```python
from build123d import *

# Parameters (mm, degrees)
SKETCH1_R               = 20
SKETCH1_R_2             = 1.475
BOSS_EXTRUDE1_DEPTH     = 6
CUT_EXTRUDE1_REACH      = 30.914
CUT_EXTRUDE1_END_RADIUS = 20
SKETCH2_R               = 1.975


with BuildPart() as part:
    # Sketch1 → Boss-Extrude1 (new body)
    # profile 1 of 2: a face of its own
    with BuildSketch(Plane.XY):
        Circle(SKETCH1_R)
        with Locations((-10.606601718, -10.606601718)):
            Circle(SKETCH1_R_2, mode=Mode.SUBTRACT)
        with Locations((10.606601718, -10.606601718)):
            Circle(SKETCH1_R_2, mode=Mode.SUBTRACT)
        with Locations((-10.606601718, 10.606601718)):
            Circle(SKETCH1_R_2, mode=Mode.SUBTRACT)
        with BuildLine():
            ThreePointArc((4.125, 0), (-1.684302549, -3.765468088), (-2.749545417, 3.075))
            ThreePointArc((-2.749545417, 3.075), (0, 4.125), (2.749545417, 3.075))
            ThreePointArc((2.749545417, 3.075), (3.765468088, 1.684302549), (4.125, 0))
        make_face(mode=Mode.SUBTRACT)
        with Locations((10.606601718, 10.606601718)):
            Circle(SKETCH1_R_2, mode=Mode.SUBTRACT)
    # profile 2 of 2: a face of its own
    with BuildSketch(Plane.XY):
        with BuildLine():
            ThreePointArc((2.749545417, 3.075), (0, 4.125), (-2.749545417, 3.075))
            Line((-2.749545417, 3.075), (2.749545417, 3.075))
        make_face()
    extrude(amount=BOSS_EXTRUDE1_DEPTH)

    # Cut-Extrude1: up to this cylinder (the profile starts inside it)
    cut_extrude1_end = Plane(origin=(0, 0, 3), z_dir=(0, 0, -1)) * Cylinder(CUT_EXTRUDE1_END_RADIUS, 102.828, mode=Mode.PRIVATE)
    # Sketch2 → Cut-Extrude1 (cut, up to the surface)
    with BuildSketch(Plane(origin=(0, 0, 0), x_dir=(1, 0, 0), z_dir=(0, 1, 0)), mode=Mode.PRIVATE) as cut_extrude1_sk1:
        with Locations(Location((0, -3, 0), (0, 0, 90))):
            Circle(SKETCH2_R)
    cut_extrude1_tool1 = extrude(cut_extrude1_sk1.sketch, amount=CUT_EXTRUDE1_REACH, mode=Mode.PRIVATE) & cut_extrude1_end
    add(cut_extrude1_tool1.solids().sort_by_distance((0, 0, 3))[0], mode=Mode.SUBTRACT)


solid = part.part
```
Design review of the part built by this model. Coordinates are the model's own, in mm. A direction names the side the tool comes from. Coordinates: 2 decimals unless noted, no trailing zeros. Loops run counter-clockwise (first coordinate to the right, second up) from the corner with the lowest first, then second, coordinate; pieces in that order, holes last.
Q1. For pin 1 (2.5 mm diameter, centred on x = 0, z = 2, fed in from -Y); pin 2 (1 mm diameter, centred on y = 5, z = 2.5, fed in from +X); pin 3 (3.5 mm diameter, centred on x = 0, z = 3, fed in from +Y), all flat-tipped, find the tip position at first contact; note any pin that passes through.
Reported:
pin 1: stops at y = -20
pin 2: stops at x = 19.49
pin 3: stops at y = -3.74
Q2. We need section B-B on z = 4. State the section outline as (x, y) points (3 decimals), and give its area (3 significant figures).
Reported:
outline: (-2.75, 3.075) - (-1.703, 3.075) - (-1.703, 19.927) arc R20 ccw (long way) to (1.703, 19.927) - (1.703, 3.075) - (2.75, 3.075) arc R4.125 cw (long way) to start; hole circle Ø2.95 at (-10.607, -10.607); hole circle Ø2.95 at (-10.607, 10.607); hole circle Ø2.95 at (10.607, -10.607); hole circle Ø2.95 at (10.607, 10.607)
area: 1,120 mm2
Q3. We need section D-D on x = -16. State the section outline as (y, z) points.
Reported:
outline: (-12, 0) - (12, 0) - (12, 6) - (-12, 6) - close
Q4. To check wall thickness, follow line 1 (Y direction, x = 11.5, z = 4); line 2 (X direction, y = 9.5, z = 5.75); line 3 (Y direction, x = 11, z = 2.75). State the ranges of each line that lie inside material, in increasing order.
Reported:
line 1: y = -16.36 to -11.78, -9.43 to 9.43, 11.78 to 16.36
line 2: x = -17.6 to -11.58, -9.63 to 9.63, 11.58 to 17.6
line 3: y = -16.7 to -12.03, -9.19 to 9.19, 12.03 to 16.7
Q5. We need section C-C on y = 14. State the section outline as (x, z) points (3 decimals).
Reported:
outline: (-14.283, 0) - (14.283, 0) - (14.283, 6) - (-14.283, 6) - close; hole circle Ø3.95 at (0, 3)
Q6. Tool access review of faces 5 (the face through (0, 5, 0)), 6 (the face through (-2, 3.075, 2)), 7 (the face through (1.2, 11.42, 4.57)): name each direction out of +Z, -Z, +X, -X, +Y, -Y from which nothing blocks a thin tool from reaching the whole face with its end or side.
Reported:
face 5: -Z, +X, -X, +Y, -Y
face 6: +Z, -Z
face 7: +Y
Q7. We need section A-A on x = 0. State the section outline as (y, z) points (3 decimals), and give its area (3 significant figures).
Reported:
outline: (-20, 0) - (-4.125, 0) - (-4.125, 6) - (-20, 6) - close; (3.075, 0) - (20, 0) - (20, 1.025) - (3.075, 1.025) - close; (3.075, 4.975) - (20, 4.975) - (20, 6) - (3.075, 6) - close
area: 130 mm2
Q8. The part is to be moulded in two halves that separate along X. For faces 1 (the face through (0, 5, 6)), 2 (the face through (-4.336, -19.524, 2.958)), 3 (the face through (-11.78, 9.71, 2.96)), 4 (the face through (10.287, 9.167, 2.958)), say which applies: +X half, -X half, draft (parallel to the pull), parting line (faces both ways), or undercut.
Reported:
face 1: draft
face 2: parting line
face 3: undercut
face 4: undercut
